Can you work these out from the model? Positions are in its coordinate system, mm. Give positions to 0.01 mm unless a question says otherwise; leave off trailing zeros. Order: outer loops, then holes, each group sorted by start corner. A loop starts at its lowest first (then second) coordinate and runs counter-clockwise, first axis right, second up. Notation, with made-up numbers: (11.5, 83.5) -> (55.5, 83.5) arc R16 ccw to (55.5, 102.5) -> close; hole circle Ø8 at (63.25, 11.25). An arc over 180 degrees is marked (long way). Answer as a JSON object with one key per item and string values.
```python
from build123d import *

# Parameters (mm, degrees)
ESTRUSIONE_ESTRUSIONE1_DEPTH = 5
SCHIZZO2_R                   = 4
SCHIZZO2_R_2                 = 1.5
TAGLIO_ESTRUSIONE1_DEPTH     = 6


with BuildPart() as part:
    # Schizzo3 → Estrusione-Estrusione1 (new body)
    with BuildSketch(Plane(origin=(0, 0, 0), x_dir=(0, 0, -1), z_dir=(1, 0, 0))):
        with BuildLine():
            Line((40.160183768, 51.647051924), (40.160183768, 100.394835388))
            Line((40.160183768, 100.394835388), (12.334616938, 111.608123513))
            ThreePointArc((12.334616938, 111.608123513), (-5.305430843, 113.570729245), (-21.410737295, 106.111358555))
            Line((-21.410737295, 106.111358555), (-44.239245072, 86.647051924))
            Line((-44.239245072, 86.647051924), (-44.239245072, 51.647051924))
            Line((-44.239245072, 51.647051924), (40.160183768, 51.647051924))
        make_face()
    extrude(amount=ESTRUSIONE_ESTRUSIONE1_DEPTH)

    # Schizzo2 → Taglio-Estrusione1 (cut, through all)
    with BuildSketch(Plane(origin=(0, 0, 0), x_dir=(0, 0, -1), z_dir=(1, 0, 0))):
        with Locations((-95, 0)):
            Circle(SCHIZZO2_R)
        with Locations((201, 0)):
            Circle(SCHIZZO2_R)
        with Locations((0, 101)):
            Circle(SCHIZZO2_R_2)
        with Locations((0, 61)):
            Circle(SCHIZZO2_R_2)
        with Locations((20, 81)):
            Circle(SCHIZZO2_R_2)
        with Locations((-20, 81)):
            Circle(SCHIZZO2_R_2)
        with Locations((0, 81)):
            Circle(SCHIZZO2_R)
    extrude(amount=TAGLIO_ESTRUSIONE1_DEPTH, mode=Mode.SUBTRACT)


solid = part.part
```
1. Please list where these lines run through material, in increasing order: L1, parallel to Z at x = 2, y = 81; L2, parallel to Y at x = 1.15, z = 0; L3, parallel to Z at x = 3.75, y = 78.
Worked answers:
{"L1": "-40.16 to -21.5, -18.5 to -4, 4 to 18.5, 21.5 to 44.24", "L2": "51.65 to 59.5, 62.5 to 77, 85 to 99.5, 102.5 to 114", "L3": "-40.16 to -2.65, 2.65 to 44.24"}
2. Will these pins go through, and if not, where does the flat tip stop? pin 1 Ø4 at (y, z) = (81, -20) entering from +X; pin 2 Ø1 at (x, z) = (3.5, -8.5) entering from +Y.
Worked answers:
{"pin 1": "x = 5", "pin 2": "y = 113.02"}
3. If we section it at C-C on x = 1.8: Please give me the cut outline in (y, z).
Worked answers:
{"outline": "(51.65, -40.16) -> (100.39, -40.16) -> (111.61, -12.33) arc R33 ccw to (106.11, 21.41) -> (86.65, 44.24) -> (51.65, 44.24) -> close; hole circle Ø3 at (61, 0); hole circle Ø8 at (81, 0); hole circle Ø3 at (81, -20); hole circle Ø3 at (81, 20); hole circle Ø3 at (101, 0)"}
4. If we section it at D-D on y = 81: Please give me the cut outline in (x, z), then the cut area to 3 significant figures.
Worked answers:
{"outline": "(0, -40.16) -> (5, -40.16) -> (5, -21.5) -> (0, -21.5) -> close; (0, -18.5) -> (5, -18.5) -> (5, -4) -> (0, -4) -> close; (0, 4) -> (5, 4) -> (5, 18.5) -> (0, 18.5) -> close; (0, 21.5) -> (5, 21.5) -> (5, 44.24) -> (0, 44.24) -> close", "area": "352 mm²"}
5. If we section it at B-B on z = 0: Please give me the cut outline in (x, y), then the cut area to 3 significant figures.
Worked answers:
{"outline": "(0, 51.65) -> (5, 51.65) -> (5, 59.5) -> (0, 59.5) -> close; (0, 62.5) -> (5, 62.5) -> (5, 77) -> (0, 77) -> close; (0, 85) -> (5, 85) -> (5, 99.5) -> (0, 99.5) -> close; (0, 102.5) -> (5, 102.5) -> (5, 114) -> (0, 114) -> close", "area": "242 mm²"}
6. If we section it at A-A on y = 61: Please give me the cut outline in (x, z), then the cut area to 3 significant figures.
Worked answers:
{"outline": "(0, -40.16) -> (5, -40.16) -> (5, -1.5) -> (0, -1.5) -> close; (0, 1.5) -> (5, 1.5) -> (5, 44.24) -> (0, 44.24) -> close", "area": "407 mm²"}
7. If we mould it in two halves opening along Z, with no side actions, what happens to faces 1 (the face through (2.465, 102.487, 0.195)), 2 (the face through (2, 76, -40.16)), 3 (the face through (5, 76, 3))? For each: +Z half, -Z half, draft (parallel to the pull), parting line (faces both ways), or undercut.
Worked answers:
{"face 1": "undercut", "face 2": "-Z half", "face 3": "draft"}
